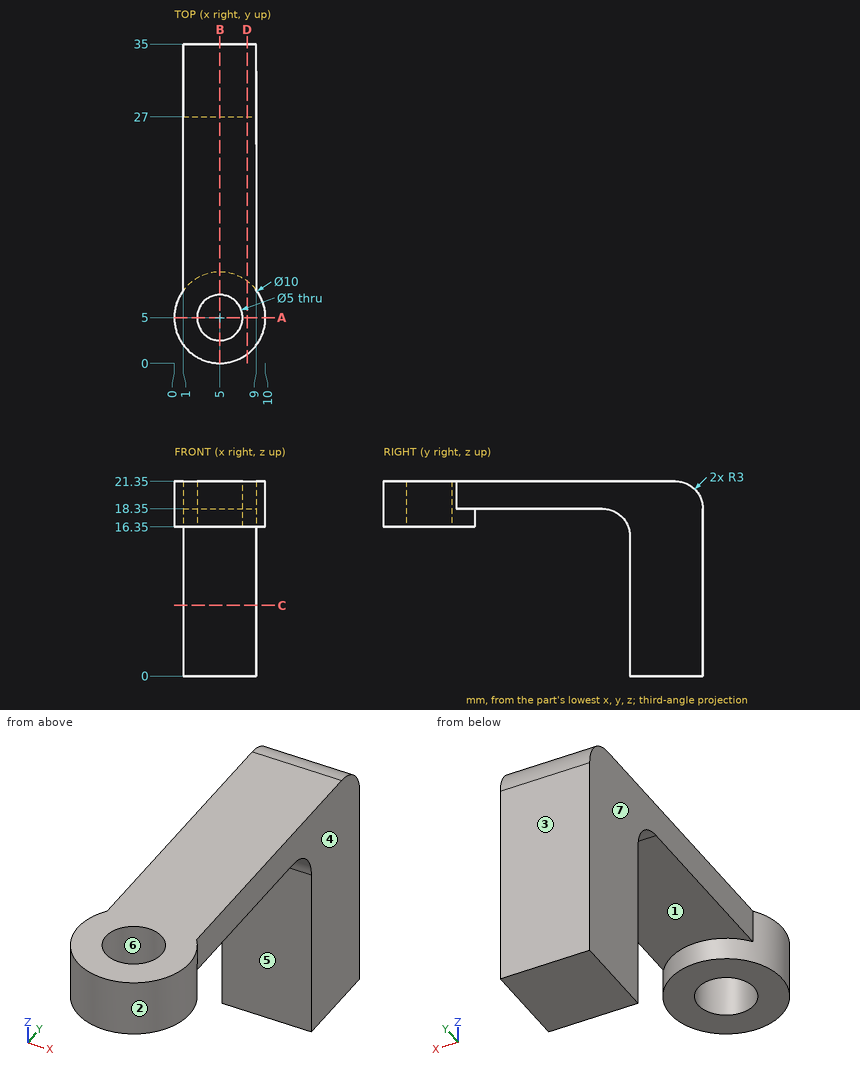
Geometry check sheet. Reference: drawing and pictorial views, mm from the part's lowest x, y, z. A direction names the side the tool comes from. Round coordinates to 2 decimals unless told otherwise and drop trailing zeros. Loops run counter-clockwise (first coordinate to the right, second up) from the corner with the lowest first, then second, coordinate; pieces in that order, holes last. Notation, with made-up numbers: (43, -25) - (51, -25) arc R25 cw to (51, 12) - close; hole circle Ø10 at (8, -20). An arc over 180 degrees is marked (long way). Write item = value, one per line. Start each with the question number.
Q1. Thickness scan on L1, parallel to Z at x = 4, y = 20.5; L2, parallel to Y at x = 8, z = 18; L3, parallel to Y at x = 5, z = 19. Record the ranges inside material, lowest first.
Q2. Section check D-D (x = 8). Record the boundary of the cut face in (y, z).
Q3. Access from +Z, -Z, +X, -X, +Y, -Y to the whole of each face (thin tool, end or side, straight path). Record for the marked faces 5, 6 and 7.
Q4. Section check B-B (x = 5). Record the boundary of the cut face in (y, z), plus the area to 3 significant figures.
Q5. Depth check by flat-ended pin: P1, Ø2.5, axis at x = 5, y = 17.5, coming from the -Z side; P2, Ø10, axis at y = 25, z = 18, coming from the -X side; P3, Ø1.5, axis at x = 9, z = 14.5, coming from the -Y side; P4, Ø6.5, axis at y = 22.5, z = 14.5, coming from the -X side. Enter the tip coordinate at first touch or a pass-through.
Q6. Section check C-C (z = 7.75). Record the boundary of the cut face in (x, y), plus the area to 3 significant figures.
Q7. Release check for a two-part mould opening along Y. For the marked faces 1, 2, 3 and 4 record: pulls with the +Y half, pulls with the -Y half, needs draft (parallel to the pull), parting line crosses it, or undercut.
Q8. Section check A-A (y = 5). Record the boundary of the cut face in (x, z), plus the area to 3 significant figures.
Derived:
q1.L1 = 18.35 to 21.35
q1.L2 = 1 to 9, 25.41 to 35
q1.L3 = 0 to 2.5, 7.5 to 34.93
q2.outline = (1, 16.35) - (9, 16.35) - (9, 18.35) - (24, 18.35) arc R3 cw to (27, 15.35) - (27, 0) - (35, 0) - (35, 18.35) arc R3 ccw to (32, 21.35) - (1, 21.35) - close
q3.face_5 = -Z, +X, -X, -Y
q3.face_6 = +Z, -Z
q3.face_7 = +Z, -Z, -X, +Y
q4.outline = (0, 16.35) - (2.5, 16.35) - (2.5, 21.35) - (0, 21.35) - close; (7.5, 16.35) - (10, 16.35) - (10, 18.35) - (24, 18.35) arc R3 cw to (27, 15.35) - (27, 0) - (35, 0) - (35, 18.35) arc R3 ccw to (32, 21.35) - (7.5, 21.35) - close
q4.area = 247 mm^2
q5.P1 = 18.35
q5.P2 = 1
q5.P3 = 27
q5.P4 = through
q6.outline = (1, 27) - (9, 27) - (9, 35) - (1, 35) - close
q6.area = 64.0 mm^2
q7.face_1 = undercut
q7.face_2 = undercut
q7.face_3 = pulls with the +Y half
q7.face_4 = needs draft
q8.outline = (0, 16.35) - (2.5, 16.35) - (2.5, 21.35) - (0, 21.35) - close; (7.5, 16.35) - (10, 16.35) - (10, 21.35) - (7.5, 21.35) - close
q8.area = 25.0 mm^2
